```python
from build123d import *

# Parameters (mm, degrees)
SKETCH_1_R               = 32
SKETCH_1_R_2             = 4
SKETCH_1_R_3             = 3
EXTRUDE_1_DEPTH          = 19
FILLET_1_R               = 2
SKETCH_2_R               = 5.375
CUT_EXTRUDE_1_DEPTH      = 15.5
SKETCH_3_R               = 2.625
CUT_EXTRUDE_2_DEPTH      = 15
SKETCH_4_R               = 1.25
CUT_EXTRUDE_3_DEPTH      = 50.081564832
SKETCH_7_R               = 1.95
CUT_EXTRUDE_5_DEPTH      = 3
CHAMFER_1_SIZE           = 1
SKETCH_8_R               = 7.25
CUT_EXTRUDE_6_DEPTH      = 10
SKETCH_9_R               = 0.75
CUT_EXTRUDE_7_DEPTH      = 50.081564832
CUT_EXTRUDE_9_REACH      = 76.034
CUT_EXTRUDE_9_END_RADIUS = 2.625
SKETCH_11_R              = 0.9
PATTERN_CIRCULAR_7_COUNT = 3


with BuildPart() as part:
    # Эскиз1 → Бобышка-Вытянуть1 (new body)
    with BuildSketch(Plane(origin=(0, 0, 0), x_dir=(1, 0, 0), z_dir=(0, 1, 0))):
        with Locations(Location((0, 0, 0), (0, 0, 270))):
            Circle(SKETCH_1_R)
        with Locations(Location((0, 0, 0), (0, 0, 270))):
            Circle(SKETCH_1_R_2, mode=Mode.SUBTRACT)
        with Locations(Location((0, 25, 0), (0, 0, 270))):
            Circle(SKETCH_1_R_3, mode=Mode.SUBTRACT)
        with Locations(Location((21.650635095, -12.5, 0), (0, 0, 270))):
            Circle(SKETCH_1_R_3, mode=Mode.SUBTRACT)
        with Locations(Location((-21.650635095, -12.5, 0), (0, 0, 270))):
            Circle(SKETCH_1_R_3, mode=Mode.SUBTRACT)
    extrude(amount=EXTRUDE_1_DEPTH)

    # Скругление1
    fillet_1_edges = [part.edges().sort_by_distance(p)[0] for p in [
        (0, 0, -32),
    ]]
    fillet(fillet_1_edges, radius=FILLET_1_R)

    # Эскиз2 → Вырез-Вытянуть1 (cut)
    with BuildSketch(Plane(origin=(0, 19, 0), x_dir=(1, 0, 0), z_dir=(0, 1, 0))):
        with Locations(Location((0, 25, 0), (0, 0, 270))):
            Circle(SKETCH_2_R)
        with Locations(Location((21.650635095, -12.5, 0), (0, 0, 270))):
            Circle(SKETCH_2_R)
        with Locations(Location((-21.650635095, -12.5, 0), (0, 0, 270))):
            Circle(SKETCH_2_R)
    extrude(amount=-CUT_EXTRUDE_1_DEPTH, mode=Mode.SUBTRACT)

    # Эскиз3 → Вырез-Вытянуть2 (cut)
    with BuildSketch(Plane.XZ):
        with Locations(Location((0, 25, 0), (0, 0, 270))):
            Circle(SKETCH_3_R)
        with Locations(Location((21.650635095, -12.5, 0), (0, 0, 270))):
            Circle(SKETCH_3_R)
        with Locations(Location((-21.650635095, -12.5, 0), (0, 0, 270))):
            Circle(SKETCH_3_R)
    extrude(amount=-CUT_EXTRUDE_2_DEPTH, mode=Mode.SUBTRACT)

    # Эскиз4 → Вырез-Вытянуть3 (cut, through all)
    with BuildSketch(Plane(origin=(0, 19, 0), x_dir=(1, 0, 0), z_dir=(0, 1, 0))):
        with Locations(Location((0, 10, 0), (0, 0, 270))):
            Circle(SKETCH_4_R)
        with Locations(Location((8.660254038, 5, 0), (0, 0, 270))):
            Circle(SKETCH_4_R)
        with Locations(Location((8.660254038, -5, 0), (0, 0, 270))):
            Circle(SKETCH_4_R)
        with Locations(Location((0, -10, 0), (0, 0, 270))):
            Circle(SKETCH_4_R)
        with Locations(Location((-8.660254038, -5, 0), (0, 0, 270))):
            Circle(SKETCH_4_R)
        with Locations(Location((-8.660254038, 5, 0), (0, 0, 270))):
            Circle(SKETCH_4_R)
    extrude(amount=-CUT_EXTRUDE_3_DEPTH, mode=Mode.SUBTRACT)

    # Эскиз7 → Вырез-Вытянуть5 (cut)
    with BuildSketch(Plane.XZ):
        with Locations(Location((8.660254038, 5, 0), (0, 0, 270))):
            Circle(SKETCH_7_R)
        with Locations(Location((0, -10, 0), (0, 0, 270))):
            Circle(SKETCH_7_R)
        with Locations(Location((-8.660254038, 5, 0), (0, 0, 270))):
            Circle(SKETCH_7_R)
    extrude(amount=-CUT_EXTRUDE_5_DEPTH, mode=Mode.SUBTRACT)

    # Фаска1
    chamfer_1_edges = [part.edges().sort_by_distance(p)[0] for p in [
        (21.650635095, 0, 9.5),
        (-21.650635095, 0, 9.5),
        (0, 0, 27.625),
        (21.650635095, 0, -9.875),
        (-21.650635095, 0, -9.875),
        (0, 0, -4),
        (0, 0, -28),
    ]]
    chamfer(chamfer_1_edges, length=CHAMFER_1_SIZE)

    # Эскиз8 → Вырез-Вытянуть6 (cut)
    with BuildSketch(Plane(origin=(0, 19, 0), x_dir=(1, 0, 0), z_dir=(0, 1, 0))):
        with Locations(Location((0, 0, 0), (0, 0, 270))):
            Circle(SKETCH_8_R)
    extrude(amount=-CUT_EXTRUDE_6_DEPTH, mode=Mode.SUBTRACT)

    # Эскиз9 → Вырез-Вытянуть7 (cut, through all)
    with BuildSketch(Plane(origin=(0, 19, 0), x_dir=(1, 0, 0), z_dir=(0, 1, 0))):
        with Locations(Location((-8, 23.685438565, 0), (0, 0, 270))):
            Circle(SKETCH_9_R)
        with Locations(Location((8, 23.685438565, 0), (0, 0, 270))):
            Circle(SKETCH_9_R)
        with Locations(Location((16.512191497, -18.770922513, 0), (0, 0, 270))):
            Circle(SKETCH_9_R)
        with Locations(Location((24.512191497, -4.914516052, 0), (0, 0, 270))):
            Circle(SKETCH_9_R)
        with Locations(Location((-24.512191497, -4.914516052, 0), (0, 0, 270))):
            Circle(SKETCH_9_R)
        with Locations(Location((-16.512191497, -18.770922513, 0), (0, 0, 270))):
            Circle(SKETCH_9_R)
    extrude(amount=-CUT_EXTRUDE_7_DEPTH, mode=Mode.SUBTRACT)

    # Вырез-Вытянуть9: up to this cylinder (the profile starts outside it)
    cut_extrude_9_end = Plane(origin=(0, 9.5, 25), z_dir=(0, -1, 0)) * Cylinder(CUT_EXTRUDE_9_END_RADIUS, 158.318, mode=Mode.PRIVATE)
    # Эскиз11 → Вырез-Вытянуть9 (cut, up to the surface)
    with BuildSketch(Plane.XY.offset(32), mode=Mode.PRIVATE) as cut_extrude_9_sk1:
        with Locations((0, 9.5)):
            Circle(SKETCH_11_R)
    cut_extrude_9_tool1 = extrude(cut_extrude_9_sk1.sketch, amount=-CUT_EXTRUDE_9_REACH, mode=Mode.PRIVATE) - cut_extrude_9_end
    cut_extrude_9 = cut_extrude_9_tool1.solids().sort_by_distance((0, 9.5, 32))[0]
    add(cut_extrude_9, mode=Mode.SUBTRACT)

    # Круговой массив7: Вырез-Вытянуть9 ×3 about axis
    pattern_circular_7_axis = Axis((0, 19, 0), (0, -1, 0))
    for i in range(1, PATTERN_CIRCULAR_7_COUNT):
        add(cut_extrude_9.rotate(pattern_circular_7_axis, i * 360 / PATTERN_CIRCULAR_7_COUNT), mode=Mode.SUBTRACT)


solid = part.part
```
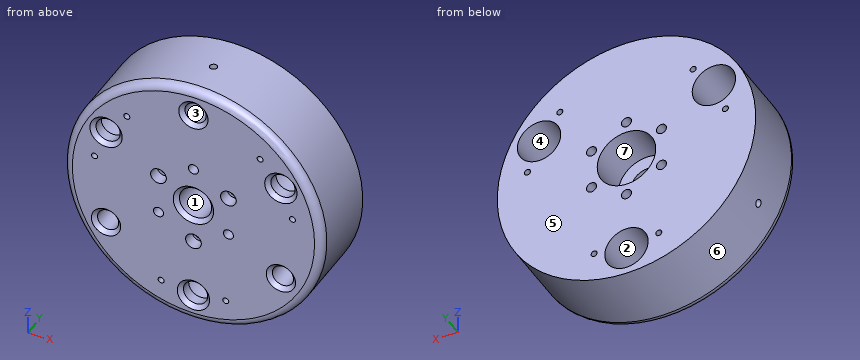
Here's how the part is built. I have some questions about the finished solid (model axes, mm). Face numbers are marked on the shaded views. A direction names the side the tool comes from. Coordinates: 2 decimals unless noted, no trailing zeros. Order: outer loops, then holes, each group sorted by start corner. A loop starts at its lowest first (then second) coordinate and runs counter-clockwise, first axis right, second up.
1) We'd pull the mould along Z, two halves only. Please class the marked faces 4, 5, 6 and 7: +Z half, -Z half, draft (parallel to the pull), parting line (faces both ways), or undercut.
2) Will these pins go through, and if not, where does the flat tip stop? pin 1 (3 mm diameter, centred on x = 23, z = 10, fed in from +Y); pin 2 (6 mm diameter, centred on x = 6.5, y = 3.5, fed in from -Z); pin 3 (1.6 mm diameter, centred on x = 1, z = 25, fed in from -Y); pin 4 (12.5 mm diameter, centred on x = 21.65, z = 12.5, fed in from -Y).
3) Imagine slicing it at B-B on y = 17.5. State how many separate pieces and enclosed holes the cut face has, and give its area (3 significant figures).
4) Imagine slicing it at A-A on z = 0. List the corners of the cut face in (x, y) for me, and give its area (3 significant figures).
5) I need wall thicknesses on line 1 (X direction, y = 14.75, z = 0); line 2 (X direction, y = 2.4, z = 12.5); line 3 (X direction, y = 10.5, z = 5). Which ranges of each line are inside material? Lowest first, please.
6) Which directions (+Z, -Z, +X, -X, +Y, -Y) give clear straight access to the entire face, cutting with the end or side of a thin tool? Please do the marked faces 1, 2 and 3.
Response values:
1. face 4: undercut
1. face 5: draft
1. face 6: parting line
1. face 7: undercut
2. pin 1: stops at y = 3.5
2. pin 2: stops at z = -31.81
2. pin 3: stops at y = 15
2. pin 4: stops at y = 0
3. separate pieces: 1
3. enclosed holes: 16
3. area: 2,740 mm2
4. outline: (-32, 2) arc R2 ccw to (-30, 0) - (-5, 0) - (-4, 1) - (-4, 9) - (-7.25, 9) - (-7.25, 19) - (-32, 19) - close; (4, 1) - (5, 0) - (30, 0) arc R2 ccw to (32, 2) - (32, 19) - (7.25, 19) - (7.25, 9) - (4, 9) - close
4. area: 996 mm2
5. line 1: x = -32 to -7.25, 7.25 to 32
5. line 2: x = -29.46 to -24.65, -18.65 to 18.65, 24.65 to 29.46
5. line 3: x = -31.61 to -25.26, -23.77 to -9.91, -7.41 to -5.25, 5.25 to 7.41, 9.91 to 23.77, 25.26 to 31.61
6. face 1: +Y, -Y
6. face 2: +Y
6. face 3: -Y
